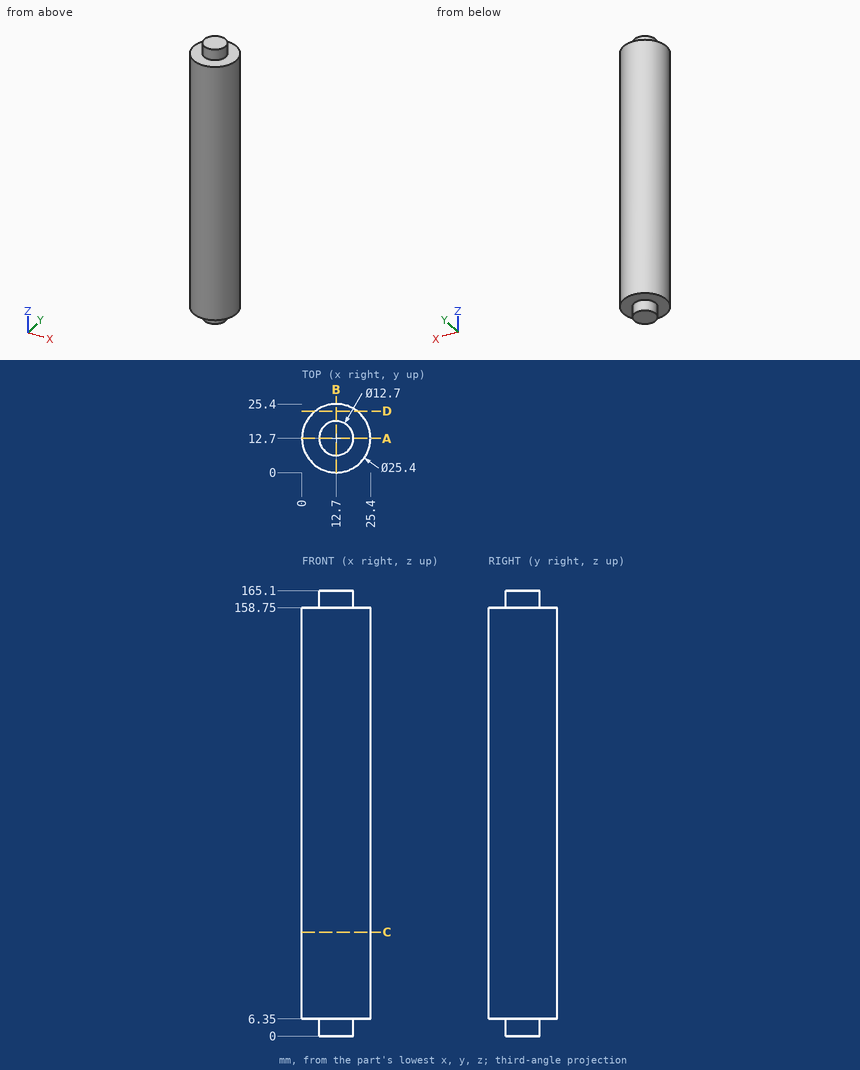
For this review, use the dimensioned drawing (mm, ordinates from the lowest corner) and the shaded views. Coordinates: 2 decimals unless noted, no trailing zeros. Loops run counter-clockwise (first coordinate to the right, second up) from the corner with the lowest first, then second, coordinate; pieces in that order, holes last.
1. Add section A-A, the plane y = 12.7. Give the boundary of the cut face in (x, z).
2. For line 1 (Y direction, x = 13.5, z = 50); line 2 (Z direction, x = 6, y = 21.75); line 3 (X direction, y = 4.75, z = 59.5), list the stretches that pass through material, from the lowest coordinate up.
3. Add section D-D, the plane y = 22.75. Give the boundary of the cut face in (x, z).
4. Add section C-C, the plane z = 38.5. Give the boundary of the cut face in (x, y).
5. Insertion check: P1, Ø12, axis at y = 4, z = 57, coming from the -X side; P2, Ø3, axis at y = 5, z = 89, coming from the +X side; P3, Ø2, axis at y = 5.5, z = 122.5, coming from the -X side. Each pin has a flat end and moves straight along its axis. Give the tip position at first contact, or say it passes through.
Result:
1. outline: (0, 6.35) - (6.35, 6.35) - (6.35, 0) - (19.05, 0) - (19.05, 6.35) - (25.4, 6.35) - (25.4, 158.75) - (19.05, 158.75) - (19.05, 165.1) - (6.35, 165.1) - (6.35, 158.75) - (0, 158.75) - close
2. line 1: y = 0.03 to 25.37
2. line 2: z = 6.35 to 158.75
2. line 3: x = 2.8 to 22.6
3. outline: (4.94, 6.35) - (20.46, 6.35) - (20.46, 158.75) - (4.94, 158.75) - close
4. outline: circle Ø25.4 at (12.7, 12.7)
5. P1: stops at x = 0.29
5. P2: stops at x = 23.78
5. P3: stops at x = 1.62
